```python
from build123d import *

# Parameters (mm, degrees)
SKETCH1_R           = 52.5
SKETCH1_R_2         = 39.5
BOSS_EXTRUDE1_DEPTH = 3
SKETCH2_R           = 1.65
CUT_EXTRUDE1_DEPTH  = 75.306796459
SKETCH3_R           = 2.5
CUT_EXTRUDE2_DEPTH  = 2
CUT_EXTRUDE3_DEPTH  = 2.5


with BuildPart() as part:
    # Sketch1 → Boss-Extrude1 (new body)
    with BuildSketch(Plane(origin=(0, 0, 0), x_dir=(1, 0, 0), z_dir=(0, 1, 0))):
        with Locations(Location((0, 0, 0), (0, 0, 270))):
            Circle(SKETCH1_R)
        with Locations(Location((0, 0, 0), (0, 0, 270))):
            Circle(SKETCH1_R_2, mode=Mode.SUBTRACT)
    extrude(amount=BOSS_EXTRUDE1_DEPTH)

    # Sketch2 → Cut-Extrude1 (cut, through all)
    with BuildSketch(Plane(origin=(0, 3, 0), x_dir=(1, 0, 0), z_dir=(0, 1, 0))):
        with Locations(Location((0, 47, 0), (0, 0, 270))):
            Circle(SKETCH2_R)
        with Locations(Location((0, -47, 0), (0, 0, 270))):
            Circle(SKETCH2_R)
        with Locations(Location((-38.500146082, 26.958092508, 0), (0, 0, 270))):
            Circle(SKETCH2_R)
        with Locations(Location((38.500146082, 26.958092508, 0), (0, 0, 270))):
            Circle(SKETCH2_R)
        with Locations(Location((38.500146082, -26.958092508, 0), (0, 0, 270))):
            Circle(SKETCH2_R)
        with Locations(Location((-38.500146082, -26.958092508, 0), (0, 0, 270))):
            Circle(SKETCH2_R)
    extrude(amount=-CUT_EXTRUDE1_DEPTH, mode=Mode.SUBTRACT)

    # Sketch3 → Cut-Extrude2 (cut)
    with BuildSketch(Plane(origin=(0, 3, 0), x_dir=(1, 0, 0), z_dir=(0, 1, 0))):
        with Locations(Location((-38.500146082, 26.958092508, 0), (0, 0, 270))):
            Circle(SKETCH3_R)
        with Locations(Location((38.500146082, 26.958092508, 0), (0, 0, 270))):
            Circle(SKETCH3_R)
        with Locations(Location((0, -47, 0), (0, 0, 270))):
            Circle(SKETCH3_R)
    extrude(amount=-CUT_EXTRUDE2_DEPTH, mode=Mode.SUBTRACT)

    # Sketch4 → Cut-Extrude3 (cut)
    with BuildSketch(Plane(origin=(0, 3, 0), x_dir=(1, 0, 0), z_dir=(0, 1, 0))):
        Polygon((-0.012280839, 49.999974863), (-2.604194862, 48.489351913), (-2.591914023, 45.48937705), (0.012280839, 44.000025137), (2.604194862, 45.510648087), (2.591914023, 48.51062295), align=None)
        Polygon((-40.07536917, -24.404923454), (-41.498866887, -27.045691193), (-39.923643798, -29.598860247), (-36.924922993, -29.511261563), (-35.501425276, -26.870493824), (-37.076648365, -24.31732477), align=None)
        Polygon((35.500146082, -26.958092508), (37.000146082, -29.55616872), (40.000146082, -29.55616872), (41.500146082, -26.958092508), (40.000146082, -24.360016297), (37.000146082, -24.360016297), align=None)
    extrude(amount=-CUT_EXTRUDE3_DEPTH, mode=Mode.SUBTRACT)


solid = part.part
```
Source: CAD feature listing. Evaluate the final solid. Frame: model axes, mm. A direction names the side the tool comes from. Round coordinates to 2 decimals unless told otherwise and drop trailing zeros. Loops run counter-clockwise (first coordinate to the right, second up) from the corner with the lowest first, then second, coordinate; pieces in that order, holes last. Notation, with made-up numbers: M -24.75,40.25 L 30.25,40.25 A25 cw 30.25,54.25 Z; hole C 40.5,30.25 d9. An arc over 180 degrees is marked long. Put each result on its own line as item: value.
(1) Section C-C, the plane y = 1.6. Return loops of the section in (x, z), and give its area (3 significant figures).
Solutions:
outline: C 0,0 d105; hole M -41.5,27.05 L -40.08,24.4 L -37.08,24.32 L -35.5,26.87 L -36.92,29.51 L -39.92,29.6 Z; hole C -38.5,-26.96 d5; hole C 0,0 d79; hole M -2.6,-48.49 L -0.01,-50 L 2.59,-48.51 L 2.6,-45.51 L 0.01,-44 L -2.59,-45.49 Z; hole C 0,47 d5; hole M 35.5,26.96 L 37,24.36 L 40,24.36 L 41.5,26.96 L 40,29.56 L 37,29.56 Z; hole C 38.5,-26.96 d5
area: 3,630 mm²
(2) Section B-B, the plane x = -17. Return loops of the section in (y, z), and give its area (3 significant figures).
Solutions:
outline: M 0,-49.67 L 3,-49.67 L 3,-35.65 L 0,-35.65 Z; M 0,35.65 L 3,35.65 L 3,49.67 L 0,49.67 Z
area: 84.1 mm²
(3) Ray query, line 1 (Z direction, x = -1.5, y = 2.1); line 2 (Z direction, x = 31.5, y = 2.95); line 3 (X direction, y = 0.6, z = 47). Return the intervals inside material, ascending. Write a range as [from, to].
Solutions:
line 1: [-52.48, -49.13], [-44.86, -39.47], [39.47, 45], [49, 52.48]
line 2: [-42, -23.83], [23.83, 42]
line 3: [-23.39, -1.65], [1.65, 23.39]
(4) Pull-direction query (Z, two-part tool) for faces 3 (the face through (1.29, 1.768, -44.745)), 4 (the face through (15.77, 1.479, 50.076)), 5 (the face through (0.07, 0.25, -48.65)); classes: released by +Z, released by -Z, zero draft, split by the parting line, or undercut.
Solutions:
face 3: undercut
face 4: split by the parting line
face 5: undercut
(5) First-contact query: pin 1 (0.8 mm diameter, centred on x = 38, y = 1, fed in from -Z); pin 2 (1 mm diameter, centred on y = 1.5, z = 11.5, fed in from +X); pin 3 (1 mm diameter, centred on y = 2, z = -34, fed in from -X). Flat tips, straight axial feed; report the tip coordinate or a pass-through.
Solutions:
pin 1: z = -36.64
pin 2: x = 51.33
pin 3: x = -40.42
(6) Access query for faces 1 (the face through (39, 2, 24.36)), 2 (the face through (-37.38, 0.51, -28.17)). Directions: +Z, -Z, +X, -X, +Y, -Y. A direction counts if a zero-diameter tool reaches every point of the face in a straight line with its end or side. Return the directions, or none.
Solutions:
face 1: +Y
face 2: +Y, -Y
(7) Section A-A, the plane z = 0. Return loops of the section in (x, y).
Solutions:
outline: M -52.5,0 L -39.5,0 L -39.5,3 L -52.5,3 Z; M 39.5,0 L 52.5,0 L 52.5,3 L 39.5,3 Z
(8) Section D-D, the plane z = 47. Return loops of the section in (x, y), and give its area (3 significant figures).
Solutions:
outline: M -23.39,0 L -1.65,0 L -1.65,1 L -2.5,1 L -2.5,3 L -23.39,3 Z; M 1.65,0 L 23.39,0 L 23.39,3 L 2.5,3 L 2.5,1 L 1.65,1 Z
area: 127 mm²
